from build123d import *

# Parameters (mm, degrees)
F0_R      = 15.875
F1_DEPTH  = 6.35
F1_FACE_R = 15.875
F3_R      = 8.382
F5_R      = 8.382
F6_DEPTH  = 12.7


with BuildPart() as f1:
    # F0 (on Right) → F1 (new body)
    with BuildSketch(Plane.YZ):
        Circle(F0_R)
    extrude(amount=F1_DEPTH)

    # F1_face (on face) → F4 section 0
    with BuildSketch(Plane.YZ.offset(6.35)):
        Circle(F1_FACE_R)
    # F3 (on offset) → F4 section 1
    with BuildSketch(Plane.YZ.offset(31.75)):
        Circle(F3_R)
    loft()

    # F5 (on face) → F6 (join)
    with BuildSketch(Plane.YZ.offset(31.75)):
        Circle(F5_R)
    extrude(amount=F6_DEPTH)


solid = f1.part
Geometry check sheet. Reference: the model listing, model coordinates, mm. Round coordinates to 2 decimals unless told otherwise and drop trailing zeros. Order: outer loops, then holes, each group sorted by start corner. A loop starts at its lowest first (then second) coordinate and runs counter-clockwise, first axis right, second up. Notation, with made-up numbers: (73.25, 89.5) - (88.25, 89.5) arc R9 cw to (88.25, 103.5) - close; hole circle Ø6 at (-33.5, -2). An arc over 180 degrees is marked (long way). One line per question, with ' | ' between items. Start each with the question number.
(1) Depth check by flat-ended pin: pin 1 Ø4 at (x, y) = (29.5, 0.5) entering from -Z; pin 2 Ø5 at (x, y) = (18, 11.5) entering from -Z; pin 3 Ø6 at (x, z) = (4.5, -11) entering from +Y. Enter the tip coordinate at first touch or a pass-through.
(2) Sectioned sample at B-B on x = 3.5. Record the cut outline in (y, z) (3 decimals).
(3) Sectioned sample at A-A on y = 0. Record the cut outline in (x, z) (3 decimals), and give its area (3 significant figures).
(4) Thickness scan on L1, parallel to Z at x = 34, y = -4.5; L2, parallel to Z at x = 30, y = -3; L3, parallel to Y at x = 39, z = -6. Record the ranges inside material, lowest first. Write a range as [from, to].
(5) Sectioned sample at C-C on x = 27. Record the cut outline in (y, z).
(6) Release check for a two-part mould opening along X. For faces 1 (the flat face through (44.45, 0, 0)), 2 (the cylindrical face through (3.131, -3.441, -15.497)), 3 (the flat face through (0, 0, 0)) record: released by +X, released by -X, zero draft, split by the parting line, or undercut.
Conclusion:
1) pin 1: stops at z = -9.63 | pin 2: stops at z = -8.79 | pin 3: stops at y = 13.71
2) outline: circle Ø31.75 at (0, 0)
3) outline: (0, -15.875) - (6.35, -15.875) - (31.75, -8.382) - (44.45, -8.382) - (44.45, 8.382) - (31.75, 8.382) - (6.35, 15.875) - (0, 15.875) - close | area: 1,030 mm2
4) L1: z = [-7.07, 7.07] | L2: z = [-8.38, 8.38] | L3: y = [-5.85, 5.85]
5) outline: circle Ø19.57 at (0, 0)
6) face 1: released by +X | face 2: zero draft | face 3: released by -X
